from build123d import *

# Parameters (mm, degrees)
SKETCH1_W           = 25.4
SKETCH1_H           = 9.525
BOSS_EXTRUDE1_DEPTH = 1.0922
BOSS_EXTRUDE2_DEPTH = 1.0922
FILLET1_R           = 1.0922
SKETCH3_R           = 0.575
CUT_EXTRUDE1_DEPTH  = 28.149190151
REVOLVE1_ANGLE      = 20
BOSS_EXTRUDE3_DEPTH = 25.4
REVOLVE2_ANGLE      = 20
BOSS_EXTRUDE4_DEPTH = 20.32
REVOLVE3_ANGLE      = 180


with BuildPart() as part:
    # Sketch1 → Boss-Extrude1 (new body)
    with BuildSketch(Plane(origin=(0, 0, 0), x_dir=(1, 0, 0), z_dir=(0, 1, 0))):
        with Locations((-12.7, -4.7625)):
            Rectangle(SKETCH1_W, SKETCH1_H)
    extrude(amount=BOSS_EXTRUDE1_DEPTH)

    # Sketch2 → Boss-Extrude2 (add)
    with BuildSketch(Plane(origin=(0, 1.0922, 0), x_dir=(1, 0, 0), z_dir=(0, 1, 0))):
        with BuildLine():
            Line((-8.128, -3.16865), (0, -3.16865))
            Line((0, -3.16865), (0, 0))
            Line((0, 0), (-25.4, 0))
            Line((-25.4, 0), (-25.4, -9.525))
            Line((-25.4, -9.525), (0, -9.525))
            Line((0, -9.525), (0, -6.35635))
            Line((0, -6.35635), (-8.128, -6.35635))
            ThreePointArc((-8.128, -6.35635), (-9.72185, -4.7625), (-8.128, -3.16865))
        make_face()
    extrude(amount=BOSS_EXTRUDE2_DEPTH)

    # Fillet1
    fillet1_edges = [part.edges().sort_by_distance(p)[0] for p in [
        (-12.7, 0, 0),
        (-12.7, 2.1844, 0),
        (-12.7, 0, 9.525),
        (-12.7, 2.1844, 9.525),
    ]]
    fillet(fillet1_edges, radius=FILLET1_R - 0.0001)  # a hair under: the kernel refuses the full size

    # Sketch3 → Cut-Extrude1 (cut, through all)
    with BuildSketch(Plane(origin=(0, 1.0922, 0), x_dir=(1, 0, 0), z_dir=(0, 1, 0))):
        with Locations(Location((-8.128, -4.7625, 0), (0, 0, 270))):
            Circle(SKETCH3_R)
        with Locations(Location((-5.528, -4.7625, 0), (0, 0, 270))):
            Circle(SKETCH3_R)
        with Locations(Location((-2.928, -4.7625, 0), (0, 0, 270))):
            Circle(SKETCH3_R)
    extrude(amount=-CUT_EXTRUDE1_DEPTH, mode=Mode.SUBTRACT)

    # Sketch5 → Revolve1 (revolve)
    with BuildSketch(Plane.ZY.offset(25.4)):
        with BuildLine():
            Line((1.0922, 0), (8.4328, 0))
            ThreePointArc((8.4328, 0), (9.205102026, 0.319897974), (9.525, 1.0922))
            ThreePointArc((9.525, 1.0922), (9.205102026, 1.864502026), (8.4328, 2.1844))
            Line((8.4328, 2.1844), (1.0922, 2.1844))
            ThreePointArc((1.0922, 2.1844), (0.319897974, 1.864502026), (0, 1.0922))
            ThreePointArc((0, 1.0922), (0.319897974, 0.319897974), (1.0922, 0))
        make_face()
    revolve(axis=Axis((-25.4, 2.1844, 9.7028), (0, 1, 0)), revolution_arc=REVOLVE1_ANGLE)

    # Sketch7 → Boss-Extrude3 (add)
    with BuildSketch(Plane(origin=(-25.547184237, 0, 9.298414632), x_dir=(0.34202014332566943, 0, 0.9396926207859082), z_dir=(-0.9396926207859082, 0, 0.34202014332566943))):
        with BuildLine():
            Line((-8.18026208, 0), (-0.83966208, 0))
            ThreePointArc((-0.83966208, 0), (0.25253792, 1.0922), (-0.83966208, 2.1844))
            Line((-0.83966208, 2.1844), (-8.18026208, 2.1844))
            ThreePointArc((-8.18026208, 2.1844), (-9.27246208, 1.0922), (-8.18026208, 0))
        make_face()
    extrude(amount=BOSS_EXTRUDE3_DEPTH)

    # Sketch9 → Revolve2 (revolve)
    with BuildSketch(Plane(origin=(-49.415376805, 0, 17.985726272), x_dir=(0.34202014332566943, 0, 0.9396926207859082), z_dir=(-0.9396926207859082, 0, 0.34202014332566943))):
        with BuildLine():
            Line((-8.18026208, 0), (-0.83966208, 0))
            ThreePointArc((-0.83966208, 0), (0.25253792, 1.0922), (-0.83966208, 2.1844))
            Line((-0.83966208, 2.1844), (-8.18026208, 2.1844))
            ThreePointArc((-8.18026208, 2.1844), (-9.27246208, 1.0922), (-8.18026208, 0))
        make_face()
    revolve(axis=Axis((-49.268192568, 2.1844, 18.39011164), (0, 1, 0)), revolution_arc=REVOLVE2_ANGLE)

    # Sketch10 → Boss-Extrude4 (add)
    with BuildSketch(Plane(origin=(-37.967124473, 0, 31.858200142), x_dir=(0.6427876096865406, 0, 0.7660444431189771), z_dir=(-0.766044443118977, 0, 0.6427876096865405))):
        with BuildLine():
            Line((-26.191940904, 0), (-18.851340904, 0))
            ThreePointArc((-18.851340904, 0), (-17.759140904, 1.0922), (-18.851340904, 2.1844))
            Line((-18.851340904, 2.1844), (-26.191940904, 2.1844))
            ThreePointArc((-26.191940904, 2.1844), (-27.284140904, 1.0922), (-26.191940904, 0))
        make_face()
    extrude(amount=BOSS_EXTRUDE4_DEPTH)

    # Sketch11 → Revolve3 (revolve)
    with BuildSketch(Plane(origin=(-53.533147557, 0, 44.919644371), x_dir=(0.6427876096865407, 0, 0.7660444431189769), z_dir=(-0.7660444431189769, 0, 0.6427876096865407))):
        with BuildLine():
            Line((-18.851340904, 2.1844), (-22.521640904, 2.1844))
            Line((-22.521640904, 2.1844), (-22.521640904, 0))
            Line((-22.521640904, 0), (-18.851340904, 0))
            ThreePointArc((-18.851340904, 0), (-17.759140904, 1.0922), (-18.851340904, 2.1844))
        make_face()
    revolve(axis=Axis((-68.00977928, 2.1844, 27.667066507), (0, -1, 0)), revolution_arc=REVOLVE3_ANGLE)


solid = part.part
Input: part model. Units: mm. Frame: model coordinates. A direction names the side the tool comes from. Give positions to 0.01 mm unless a question says otherwise; leave off trailing zeros. Use one line per item in the form item = value. Start each with the question number.
1) Set-up query: faces 1 (the cylindrical face through (-9.72, 1.63, 4.8)), 2 (the cylindrical face through (-40.49, 1.12, 4.87)). Return all of +Z, -Z, +X, -X, +Y, -Y with unobstructed straight access to the full face (end or side cutting, diameter ignored); none if empty.
2) Ray query, probe 1 along X at (y, z) = (0.5, 28); probe 2 along Z at (x, y) = (-65, 0.35); probe 3 along X at (y, z) = (0.5, 24). Return the intervals inside material, ascending. Write a range as from..to.
3) Section query B-B on y = 0.6. Count the separate pieces of the cut face and the enclosed holes in it, then the cut area to 3 significant figures.
4) Pin query (flat end, axial travel): pin 1 (3 mm diameter, centred on x = -60.5, z = 14.5, fed in from +Y); pin 2 (1.2 mm diameter, centred on y = 0.5, z = 9, fed in from -X); pin 3 (1.3 mm diameter, centred on x = -8.13, z = 4.76, fed in from +Y); pin 4 (12 mm diameter, centred on x = -65.5, z = 4, fed in from -Y). Return the tip coordinate at first contact, or that it passes through.
Outcome:
q1.face_1 = +X, +Y
q1.face_2 = -Z, -X
q2.probe_1 = -72.59..-61.27
q2.probe_2 = 19.3..30.98
q2.probe_3 = -70.78..-56.5
q3.separate_pieces = 1
q3.enclosed_holes = 3
q3.area = 724 mm^2
q4.pin_1 = 2.18
q4.pin_2 = -53.13
q4.pin_3 = 1.09
q4.pin_4 = through
